Autodesk Inventor part; units mm, degrees
ref_plane "YZ Plane" through (0, 0, 0) normal (1, 0, 0) x (0, 1, 0)
ref_plane "XZ Plane" through (0, 0, 0) normal (0, 1, 0) x (-1, 0, 0)
ref_plane "XY Plane" through (0, 0, 0) normal (0, 0, 1) x (1, 0, 0)
sketch "Sketch1" plane through (0, 0, 0) normal (0, 0, 1) x (1, 0, 0)
  line L0 (0, 0) -> (-6.35, 0)
  line L1 (-6.35, 0) -> (4.7611, 127)
  line L2 (0, 0) -> (6.35, 0)
  line L3 (6.35, 0) -> (82.55, 0) construction
  line L4 (6.35, 0) -> (28.7435, 127)
  line L5 (6.35, 0) -> (135.3092, 0) construction
  line L6 (28.7435, 127) -> (4.7611, 127)
  dimension "d0" = 6.35
  dimension "d2" = 85
  dimension "d3" = 6.35
  dimension "d6" = 80
  dimension "d9" = 127
extrude "Extrusion1" add sketch "Sketch1" along normal blind 50.8
sketch "Sketch2" plane through (4.7611, 127, 0) normal (0, 1, 0) x (1, 0, 0)
  line L0 (0, 0) -> (-11.1111, 0)
  line L1 (0, 0) -> (5.08, 0)
  line L2 (23.9825, 0) -> (0, 0)
  line L3 (5.08, 0) -> (5.08, -50.8)
  line L4 (23.9825, -50.8) -> (0, -50.8)
  line L5 (0, 0) -> (0, -50.8)
  line L6 (0, -50.8) -> (0, 0)
  point P0 (-4.7611, 0)
  dimension "d10" = 5.08
extrude "Extrusion2" add sketch "Sketch2" along normal blind 12.7
sketch "Sketch4" plane through (28.7435, 127, 50.8) normal (0, 1, 0) x (1, 0, 0)
  line L0 (0, 50.8) -> (-18.9025, 50.8)
  line L1 (0, 50.8) -> (12.7, 50.8)
  line L2 (12.7, 50.8) -> (12.7, 0)
  line L3 (0, 50.8) -> (0, 0)
  line L4 (12.7, 0) -> (0, 0)
  line L5 (-18.9025, 0) -> (-18.9025, 50.8)
  line L6 (0, 0) -> (-18.9025, 0)
  line L7 (-18.9025, 0) -> (-18.9025, 50.8)
  line L8 (-18.9025, 50.8) -> (0, 50.8)
  point P0 (-28.7435, 50.8)
  dimension "d14" = 12.7
extrude "Extrusion3" add sketch "Sketch4" against normal blind 12.7
sketch "Sketch5" plane through (9.8411, 127, 50.8) normal (0, 1, 0) x (1, 0, 0)
  line L0 (31.6025, 0) -> (31.6025, 50.8)
  line L1 (16.6631, 50.8) -> (16.6631, 0)
  circle A0 centre (20.1725, 25.4) radius 1.7526
  line L2 (31.6025, 50.8) -> (0, 50.8)
  point P0 (-9.8411, 50.8)
  dimension "d18" = 3.5052
  dimension "d19" = 11.43
  dimension "d20" = 25.4
extrude "Extrusion4" cut sketch "Sketch5" against normal blind 12.7
thread "Thread1"
properties part number "Leg-01" material "Aluminum 6061"
CAD build for the part. Positions are in the model's coordinates, mm. A direction names the side the tool comes from. Round coordinates to 2 decimals unless told otherwise and drop trailing zeros. Order: outer loops, then holes, each group sorted by start corner. A loop starts at its lowest first (then second) coordinate and runs counter-clockwise, first axis right, second up.
Item 1: Tool access for faces 1 (the face through (34, 114.3, 25)), 2 (the face through (26, 127, 25)), 3 (the face through (4.761, 133, 25)), 4 (the face through (41.444, 121, 25)), 5 (the face through (12, 71, 50.8)): list every direction of +Z, -Z, +X, -X, +Y, -Y with a clear straight run to the whole face (end or side of a thin tool).
Item 2: Mould opens along Z. For faces 6 (the face through (0, 0, 25)), 7 (the face through (12, 71, 0)), 8 (the face through (28.623, 120.739, 26.466)) say: pulls with the +Z half, pulls with the -Z half, needs draft (parallel to the pull), parting line crosses it, or undercut.
Item 3: Pin check, flat tips, straight feed: pin 1 (14 mm diameter, centred on y = 134.5, z = 31, fed in from -X); pin 2 (9.5 mm diameter, centred on x = 31.5, z = 21, fed in from +Y); pin 3 (2 mm diameter, centred on y = 103, z = 15.5, fed in from -X). Stop position of each tip, or through.
Item 4: Saw through at A-A on z = 25.4. Write the cut outline in (x, y).
Item 5: Saw through at C-C on x = 34. Write the cut outline in (y, z).
Item 6: Saw through at B-B on z = 15. Write the cut outline in (x, y), then the cut area to 3 significant figures.
Item 7: Probe line 1 along X through (y, z) = (122.75, 25.4); line 2 along Y through (x, z) = (30, 14); line 3 along X through (y, z) = (117.5, 25.4). List the from-to ranges inside material, lowest first.
Item 8: Saw through at D-D on y = 85. Write the cut outline in (x, z).
Reported:
1. face 1: +Z, -Z, +X, -Y
1. face 2: +Z, -Z, +X, +Y
1. face 3: +Z, -Z, -X, +Y
1. face 4: +Z, -Z, +X, +Y, -Y
1. face 5: +Z, +X, -X, +Y, -Y
2. face 6: needs draft
2. face 7: pulls with the -Z half
2. face 8: undercut
3. pin 1: stops at x = 4.76
3. pin 2: stops at y = 127
3. pin 3: stops at x = 2.57
4. outline: (-6.35, 0) - (6.35, 0) - (26.5, 114.3) - (28.26, 114.3) - (28.26, 127) - (9.84, 127) - (9.84, 139.7) - (4.76, 139.7) - (4.76, 127) - close; (31.77, 114.3) - (41.44, 114.3) - (41.44, 127) - (31.77, 127) - close
5. outline: (114.3, 0) - (127, 0) - (127, 50.8) - (114.3, 50.8) - close
6. outline: (-6.35, 0) - (6.35, 0) - (26.5, 114.3) - (41.44, 114.3) - (41.44, 127) - (9.84, 127) - (9.84, 139.7) - (4.76, 139.7) - (4.76, 127) - close
6. area: 2,570 mm2
7. line 1: x = 4.39 to 28.26, 31.77 to 41.44
7. line 2: y = 114.3 to 127
7. line 3: x = 3.93 to 28.26, 31.77 to 41.44
8. outline: (1.09, 0) - (21.34, 0) - (21.34, 50.8) - (1.09, 50.8) - close
